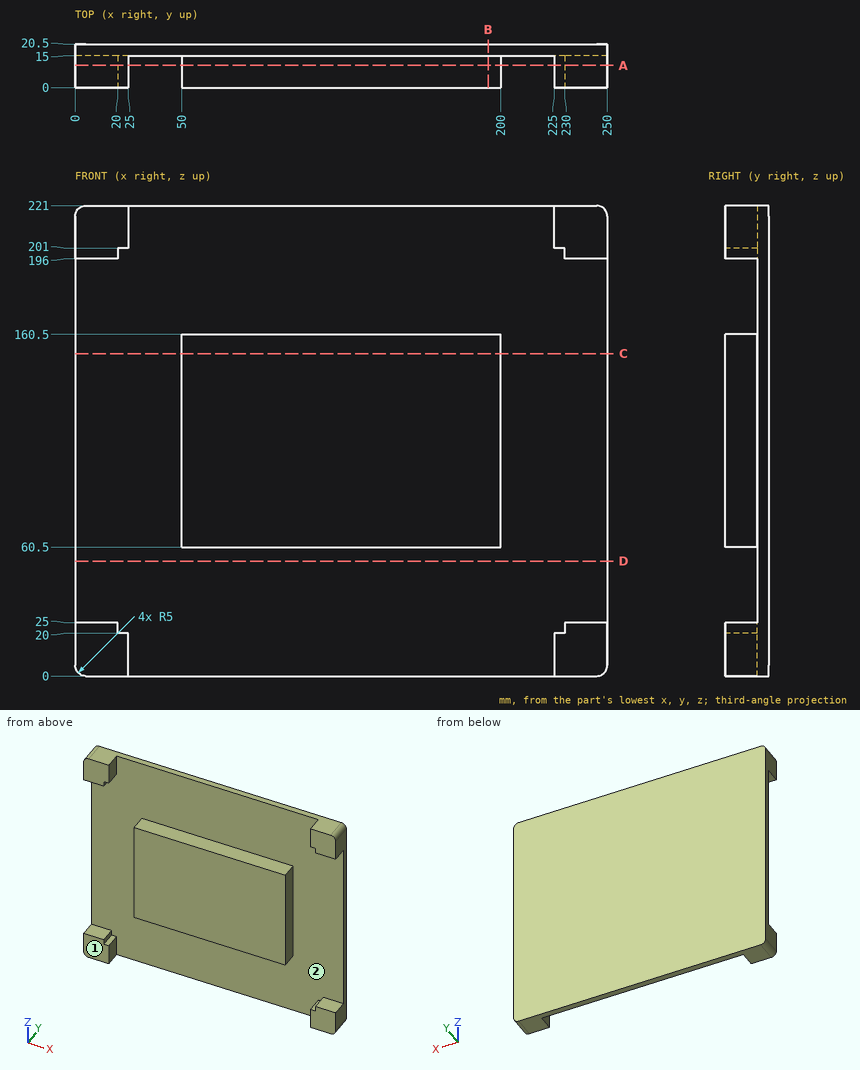
Job drawing, mm, ordinate dimensions from the low corner. One solid piece. Give positions to 0.01 mm unless a question says otherwise; leave off trailing zeros. Loops run counter-clockwise (first coordinate to the right, second up) from the corner with the lowest first, then second, coordinate; pieces in that order, holes last.
Item 1: Slice it at B-B, the plane x = 194. List the corners of the cut face in (y, z), and give its area (3 significant figures).
Answers follow:
outline: (0, 60.5) - (15, 60.5) - (15, 0) - (20.5, 0) - (20.5, 221) - (15, 221) - (15, 160.5) - (0, 160.5) - close
area: 2,720 mm2
Item 2: Pull direction X, two halves, no side cores. Call the marked faces 1 and 2: released by +X, released by -X, zero draft, split by the parting line, or undercut.
Answers follow:
face 1: zero draft
face 2: undercut
Item 3: Drill centre lines: line 1 (X direction, y = 5, z = 21.5); line 2 (Z direction, x = 72.5, y = 4.75); line 3 (X direction, y = 11.25, z = 94.5). Where is each one in solid material? Low to high.
Answers follow:
line 1: x = 0 to 20, 230 to 250
line 2: z = 60.5 to 160.5
line 3: x = 50 to 200
Item 4: Flat gauge pins, fed straight in: pin 1 (3 mm diameter, centred on y = 5, z = 104.5, fed in from +X); pin 2 (7.5 mm diameter, centred on y = 10, z = 129.5, fed in from -X); pin 3 (7.5 mm diameter, centred on x = 134, y = 8, fed in from +Z). Where does each tip first touch, or does it go through?
Answers follow:
pin 1: stops at x = 200
pin 2: stops at x = 50
pin 3: stops at z = 160.5
Item 5: Slice it at D-D, the plane z = 54. List the corners of the cut face in (x, y), and give its area (4 significant figures).
Answers follow:
outline: (0, 15) - (250, 15) - (250, 20.5) - (0, 20.5) - close
area: 1,375 mm2
Item 6: Slice it at A-A, the plane y = 10.5. Give the number of separate pieces and of enclosed holes in the cut face, and give its area (3 significant figures).
Answers follow:
separate pieces: 5
enclosed holes: 0
area: 17,400 mm2
Item 7: Slice it at C-C, the plane z = 151.5. List the corners of the cut face in (x, y).
Answers follow:
outline: (0, 15) - (50, 15) - (50, 0) - (200, 0) - (200, 15) - (250, 15) - (250, 20.5) - (0, 20.5) - close
